Can you work these out from the model? Positions are in its coordinate system, mm. A direction names the side the tool comes from. Give positions to 0.01 mm unless a question says otherwise; leave off trailing zeros. Loops run counter-clockwise (first coordinate to the right, second up) from the corner with the lowest first, then second, coordinate; pieces in that order, holes last. Notation, with made-up numbers: M 76.5,-27.5 L 127.5,-27.5 A17 cw 127.5,-23.5 Z; hole C -22,-18 d10. An arc over 180 degrees is marked long. Use CSV: the item, a comma, the result in double quotes.
Autodesk Inventor part; units mm, degrees
ref_plane "YZ Plane" through (0, 0, 0) normal (1, 0, 0) x (0, 1, 0)
sketch "Sketch2" plane through (0, 0, 0) normal (0, 0, 1) x (1, 0, 0)
  line L0 (-25.4, -12.7) -> (25.4, -12.7)
  line L1 (25.4, -12.7) -> (25.4, 12.7)
  line L2 (25.4, 12.7) -> (-25.4, 12.7)
  line L3 (-25.4, 12.7) -> (-25.4, -12.7)
  line L4 (-25.4, -12.7) -> (25.4, 12.7) construction
  line L5 (25.4, -12.7) -> (-25.4, 12.7) construction
  point P0 (0, 0)
  dimension "d4" = 50.8
  dimension "d5" = 25.4
extrude "Extrusion2" add sketch "Sketch2" along normal mid plane 38.1
sketch "Sketch3" plane through (-25.4, 12.7, 19.05) normal (0, 1, 0) x (1, 0, 0)
  line L0 (0, 0) -> (0, 38.1) construction
  line L1 (38.1, 19.05) -> (38.1, 25.908)
  line L2 (38.1, 25.908) -> (0, 25.908)
  line L3 (0, 25.908) -> (0, 19.05)
  line L4 (0, 0) -> (0, 25.4) construction
  line L5 (38.1, 19.05) -> (38.1, 12.192)
  line L6 (38.1, 12.192) -> (0, 12.192)
  line L7 (0, 12.192) -> (0, 19.05)
  line L8 (50.8, 0) -> (0, 0)
  point P0 (25.4, 19.05)
  dimension "d8" = 38.1
  dimension "d10" = 13.716
  dimension "d34" = 12.192
extrude "Extrusion3" cut sketch "Sketch3" against normal through all
sketch "Sketch4" plane through (0, 0, 19.05) normal (0, 0, 1) x (1, 0, 0)
  circle A0 centre (-12.7, 0) radius 5.2705
  line L0 (-25.4, 12.7) -> (-25.4, -12.7)
  point P0 (0, 0)
  dimension "d13" = 10.541
  dimension "d14" = 12.7
extrude "Extrusion4" cut sketch "Sketch4" against normal through all
sketch "Sketch5" plane through (25.4, -12.7, 19.05) normal (1, 0, 0) x (0, 0, -1)
  circle A0 centre (19.05, 12.7) radius 4.2164
  dimension "d27" = 8.4328
extrude "Extrusion5" cut sketch "Sketch5" against normal blind 12.7
properties part number "piston" material "PET Plastic"
Q1. I want a section at A-A, the plane x = -12.7. Please give me the cut outline in (y, z), then the cut area to 3 significant figures.
Model answer:
outline,"M -12.7,-19.05 L -5.27,-19.05 L -5.27,-6.86 L -12.7,-6.86 Z; M -12.7,6.86 L -5.27,6.86 L -5.27,19.05 L -12.7,19.05 Z; M 5.27,-19.05 L 12.7,-19.05 L 12.7,-6.86 L 5.27,-6.86 Z; M 5.27,6.86 L 12.7,6.86 L 12.7,19.05 L 5.27,19.05 Z"
area,"362 mm2"
Q2. Please list where these lines run through material, in increasing order: L1, parallel to Y at x = -12.7, z = 15.5; L2, parallel to Z at x = 2.5, y = 6.5; L3, parallel to Y at x = 22, z = 0. Write a range as from..to.
Model answer:
L1,"-12.7..-5.27, 5.27..12.7"
L2,"-19.05..-6.86, 6.86..19.05"
L3,"-12.7..-4.22, 4.22..12.7"
Q3. If we mould it in two halves opening along Y, with no side actions, what happens to faces 1 (the cylindrical face through (-17.965, 0.232, 13.039)), 2 (the flat face through (0, -12.7, -9)), 3 (the flat face through (-6, 0, -6.858))? For each: released by +Y, released by -Y, zero draft, split by the parting line, or undercut.
Model answer:
face 1,"undercut"
face 2,"released by -Y"
face 3,"zero draft"
Q4. I want a section at D-D, the plane x = -2. Please give me the cut outline in (y, z).
Model answer:
outline,"M -12.7,-19.05 L 12.7,-19.05 L 12.7,-6.86 L -12.7,-6.86 Z; M -12.7,6.86 L 12.7,6.86 L 12.7,19.05 L -12.7,19.05 Z"
Q5. I want a section at B-B, the plane z = 0. Please give me the cut outline in (x, y), then the cut area to 3 significant figures.
Model answer:
outline,"M 12.7,-12.7 L 25.4,-12.7 L 25.4,-4.22 L 12.7,-4.22 Z; M 12.7,4.22 L 25.4,4.22 L 25.4,12.7 L 12.7,12.7 Z"
area,"215 mm2"
Q6. I want a section at C-C, the plane y = 0. Please give me the cut outline in (x, z), then the cut area to 3 significant figures.
Model answer:
outline,"M -25.4,-19.05 L -17.97,-19.05 L -17.97,-6.86 L -25.4,-6.86 Z; M -25.4,6.86 L -17.97,6.86 L -17.97,19.05 L -25.4,19.05 Z; M -7.43,-19.05 L 25.4,-19.05 L 25.4,-4.22 L 12.7,-4.22 L 12.7,-6.86 L -7.43,-6.86 Z; M -7.43,6.86 L 12.7,6.86 L 12.7,4.22 L 25.4,4.22 L 25.4,19.05 L -7.43,19.05 Z"
area,"1,050 mm2"
Q7. For faces 4 (the cylindrical face through (-17.965, 0.232, -12.869)), 5 (the flat face through (-6, 0, 6.858)), which set-ups out of +Z, -Z, +X, -X, +Y, -Y let a thin tool reach every point of the face, with its end or its side?
Model answer:
face 4,"+Z, -Z"
face 5,"-X, +Y, -Y"
Q8. I'm going to push a flat-ended pin straight in: P1, Ø11, axis at y = 0, z = 0, coming from the -X side. Where does the tip first touch, or does it pass through?
Model answer:
P1,"x = 12.7"
